Source: CAD feature listing. Evaluate the final solid. Frame: model axes, mm. Give positions to 0.01 mm unless a question says otherwise; leave off trailing zeros. Loops run counter-clockwise (first coordinate to the right, second up) from the corner with the lowest first, then second, coordinate; pieces in that order, holes last. Notation, with made-up numbers: M -32,78.25 L 20,78.25 A32 cw 20,110.25 Z; hole C -7,-40 d1. An arc over 180 degrees is marked long. Put each result on its own line as item: value.
from build123d import *

# Parameters (mm, degrees)
SKETCH_1_R          = 39
EXTRUDE_1_DEPTH     = 1
SKETCH_2_R          = 1.75
CUT_EXTRUDE_1_DEPTH = 1
SKETCH_3_R          = 27.75
CUT_EXTRUDE_2_DEPTH = 1
SKETCH_4_R          = 1.75
CUT_EXTRUDE_3_DEPTH = 1
CUT_EXTRUDE_4_DEPTH = 1
CUT_EXTRUDE_5_DEPTH = 1


with BuildPart() as part:
    # 스케치1 → 보스-돌출1 (new body)
    with BuildSketch(Plane(origin=(0, 0, 0), x_dir=(1, 0, 0), z_dir=(0, 1, 0))):
        with Locations(Location((0, 0, 0), (0, 0, 270))):
            Circle(SKETCH_1_R)
    extrude(amount=EXTRUDE_1_DEPTH)

    # 스케치2 → 컷-돌출1 (cut)
    with BuildSketch(Plane(origin=(0, 1, 0), x_dir=(1, 0, 0), z_dir=(0, 1, 0))):
        with Locations(Location((29.25, 16.887495374, 0), (0, 0, 270))):
            Circle(SKETCH_2_R)
        with Locations(Location((-29.25, 16.887495374, 0), (0, 0, 270))):
            Circle(SKETCH_2_R)
        with Locations(Location((0, -33.774990748, 0), (0, 0, 270))):
            Circle(SKETCH_2_R)
    extrude(amount=-CUT_EXTRUDE_1_DEPTH, mode=Mode.SUBTRACT)

    # 스케치3 → 컷-돌출2 (cut)
    with BuildSketch(Plane(origin=(0, 1, 0), x_dir=(1, 0, 0), z_dir=(0, 1, 0))):
        with Locations(Location((0, 0, 0), (0, 0, 270))):
            Circle(SKETCH_3_R)
    extrude(amount=-CUT_EXTRUDE_2_DEPTH, mode=Mode.SUBTRACT)

    # 스케치4 → 컷-돌출3 (cut)
    with BuildSketch(Plane(origin=(0, 1, 0), x_dir=(1, 0, 0), z_dir=(0, 1, 0))):
        with Locations(Location((33.75, 13.887495374, 0), (0, 0, 270))):
            Circle(SKETCH_4_R)
        with Locations(Location((-33.75, 13.887495374, 0), (0, 0, 90))):
            Circle(SKETCH_4_R)
    extrude(amount=-CUT_EXTRUDE_3_DEPTH, mode=Mode.SUBTRACT)

    # 스케치5 → 컷-돌출4 (cut)
    with BuildSketch(Plane(origin=(0, 1, 0), x_dir=(1, 0, 0), z_dir=(0, 1, 0))):
        with BuildLine():
            Line((-41.165274156, 21.887495374), (-21.598612137, 21.887495374))
            ThreePointArc((-21.598612137, 21.887495374), (0, 30.75), (21.598612137, 21.887495374))
            Line((21.598612137, 21.887495374), (39.254048052, 21.887495374))
            Line((39.254048052, 21.887495374), (39.254048052, 46.515320785))
            Line((39.254048052, 46.515320785), (-41.165274156, 46.515320785))
            Line((-41.165274156, 46.515320785), (-41.165274156, 21.887495374))
        make_face()
    extrude(amount=-CUT_EXTRUDE_4_DEPTH, mode=Mode.SUBTRACT)

    # 스케치6 → 컷-돌출5 (cut)
    with BuildSketch(Plane(origin=(0, 1, 0), x_dir=(1, 0, 0), z_dir=(0, 1, 0))):
        Polygon((37.13022954, 19.961121964), (37.13022954, -11.930886568), (13.650716042, -36.532970746), (-13.650716042, -36.532970746), (-37.13022954, -11.930886568), (-37.13022954, 19.961121964), (-57.208624866, 19.961121964), (-57.208624866, -51.243312927), (54.097642537, -51.243312927), (54.097642537, 19.961121964), align=None)
    extrude(amount=-CUT_EXTRUDE_5_DEPTH, mode=Mode.SUBTRACT)


solid = part.part
1. Contact query for flat-ended pins moving along their axis: P1, Ø5.5, axis at x = 0, z = 33.77, coming from the +Y side; P2, Ø0.5, axis at x = 24.5, y = 0.5, coming from the -Z side. Output: stop coordinate, or through.
Found:
P1: y = 1
P2: z = -21.89
2. Section query C-C (x = 0). Output: boundary loops of the cut face in (y, z) (3 decimals).
Found:
outline: M 0,-30.75 L 1,-30.75 L 1,-27.75 L 0,-27.75 Z; M 0,27.75 L 1,27.75 L 1,32.025 L 0,32.025 Z; M 0,35.525 L 1,35.525 L 1,36.533 L 0,36.533 Z
3. Draft query along X for faces 1 (the cylindrical face through (34.28, 0.51, -12.22)), 2 (the cylindrical face through (-35.026, 0.493, -17.152)), 3 (the flat face through (3, 0, 28)). Return one class per face: pulls with the +X half, pulls with the -X half, needs draft (parallel to the pull), parting line crosses it, or undercut.
Found:
face 1: undercut
face 2: pulls with the -X half
face 3: needs draft
4. Section query B-B (y = 0.4). State how many separate pieces and enclosed holes the cut face has, plus the area to 3 significant figures.
Found:
separate pieces: 1
enclosed holes: 6
area: 1,510 mm^2
5. Material intervals for line 1 (X direction, y = 0.4, z = -16.5); line 2 (X direction, y = 0.4, z = -12); line 3 (X direction, y = 0.85, z = 9.5), sorted ascending. Write a range as from..to.
Found:
line 1: -35.34..-30.96, -27.54..-22.31, 22.31..27.54, 30.96..35.34
line 2: -37.11..-25.02, 25.02..37.11
line 3: -37.13..-26.07, 26.07..37.13
6. Section query A-A (z = 0). Output: boundary loops of the cut face in (x, y), plus the area to 3 significant figures.
Found:
outline: M -37.13,0 L -27.75,0 L -27.75,1 L -37.13,1 Z; M 27.75,0 L 37.13,0 L 37.13,1 L 27.75,1 Z
area: 18.8 mm^2
7. Section query D-D (z = -14). Output: boundary loops of the cut face in (x, y).
Found:
outline: M -36.4,0 L -35.5,0 L -35.5,1 L -36.4,1 Z; M -32,0 L -23.96,0 L -23.96,1 L -32,1 Z; M 23.96,0 L 32,0 L 32,1 L 23.96,1 Z; M 35.5,0 L 36.4,0 L 36.4,1 L 35.5,1 Z
